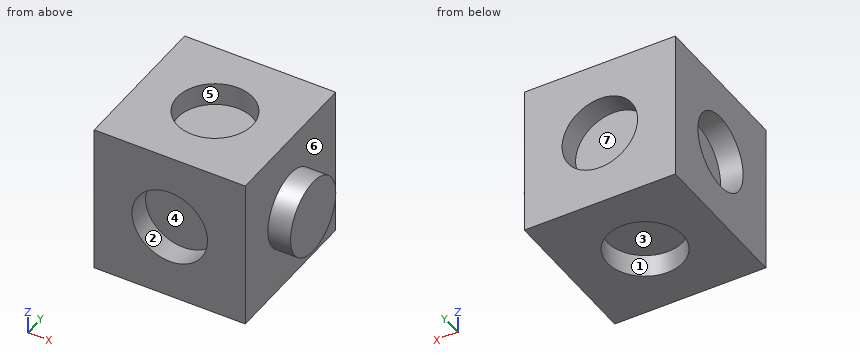
```python
from build123d import *

# Parameters (mm, degrees)
F0_W      = 25.4
F0_H      = 25.4
F1_DEPTH  = 25.4
F7_R      = 6.35
F8_DEPTH  = 3.81
F6_R      = 6.35
F9_DEPTH  = 3.81
F5_R      = 6.35
F10_DEPTH = 3.81
F4_R      = 6.35
F11_DEPTH = 3.81
F3_R      = 6.35
F12_DEPTH = 3.81
F2_R      = 6.35
F13_DEPTH = 3.81


with BuildPart() as f1:
    # F0 (on Front) → F1 (new body)
    with BuildSketch(Plane.XZ):
        with Locations((5.750718, -12.019807)):
            Rectangle(F0_W, F0_H)
    extrude(amount=F1_DEPTH)

    # F7 (on face) → F8 (cut)
    with BuildSketch(Plane(origin=(0, 0, 0), x_dir=(-1, 0, 0), z_dir=(0, 1, 0))):
        with Locations((-5.750718, -12.019807)):
            Circle(F7_R)
    extrude(amount=-F8_DEPTH, mode=Mode.SUBTRACT)

    # F6 (on face) → F9 (cut)
    with BuildSketch(Plane(origin=(-6.949282, 0, 0), x_dir=(0, -1, 0), z_dir=(-1, 0, 0))):
        with Locations((12.7, -12.019807)):
            Circle(F6_R)
    extrude(amount=-F9_DEPTH, mode=Mode.SUBTRACT)

    # F5 (on face) → F10 (cut)
    with BuildSketch(Plane.XY.offset(0.680193)):
        with Locations((5.75072, -12.7)):
            Circle(F5_R)
    extrude(amount=-F10_DEPTH, mode=Mode.SUBTRACT)

    # F4 (on face) → F11 (join)
    with BuildSketch(Plane.YZ.offset(18.450718)):
        with Locations((-12.7, -12.019807)):
            Circle(F4_R)
    extrude(amount=F11_DEPTH)

    # F3 (on face) → F12 (cut)
    with BuildSketch(Plane(origin=(0, 0, -24.719807), x_dir=(1, 0, 0), z_dir=(0, 0, -1))):
        with Locations((5.750718, 12.7)):
            Circle(F3_R)
    extrude(amount=-F12_DEPTH, mode=Mode.SUBTRACT)

    # F2 (on face) → F13 (cut)
    with BuildSketch(Plane.XZ.offset(25.4)):
        with Locations((5.750718, -12.019807)):
            Circle(F2_R)
    extrude(amount=-F13_DEPTH, mode=Mode.SUBTRACT)


solid = f1.part
```
The listing builds one solid part. Answer for the finished solid, in the listing's coordinates (mm). Face numbers are marked on the shaded views. A direction names the side the tool comes from. Give positions to 0.01 mm unless a question says otherwise; leave off trailing zeros. Order: outer loops, then holes, each group sorted by start corner. A loop starts at its lowest first (then second) coordinate and runs counter-clockwise, first axis right, second up. Notation, with made-up numbers: (87.5, -21.75) -> (107.5, -21.75) arc R21 cw to (107.5, 14.25) -> close; hole circle Ø7 at (-18.5, 38.5). An arc over 180 degrees is marked (long way). One line per item, written item: value.
1) Find section A-A, the plane y = -12.7. Determine the outline of the cut face in (x, z), plus the area to 3 significant figures.
Reported:
outline: (-6.95, -24.72) -> (-0.6, -24.72) -> (-0.6, -20.91) -> (12.1, -20.91) -> (12.1, -24.72) -> (18.45, -24.72) -> (18.45, -18.37) -> (22.26, -18.37) -> (22.26, -5.67) -> (18.45, -5.67) -> (18.45, 0.68) -> (12.1, 0.68) -> (12.1, -3.13) -> (-0.6, -3.13) -> (-0.6, 0.68) -> (-6.95, 0.68) -> (-6.95, -5.67) -> (-3.14, -5.67) -> (-3.14, -18.37) -> (-6.95, -18.37) -> close
area: 548 mm^2
2) Find section D-D, the plane y = -4.75. Determine the outline of the cut face in (x, z).
Reported:
outline: (-6.95, -24.72) -> (18.45, -24.72) -> (18.45, 0.68) -> (-6.95, 0.68) -> close
3) Determine the mould class of the marked faces 1, 2, 3 and 4 for opening direction Z: pulls with the +Z half, pulls with the -Z half, needs draft (parallel to the pull), parting line crosses it, or undercut.
Reported:
face 1: needs draft
face 2: undercut
face 3: pulls with the -Z half
face 4: undercut
4) Find section B-B, the plane z = -7.5. Determine the outline of the cut face in (x, y).
Reported:
outline: (-6.95, -25.4) -> (1.29, -25.4) -> (1.29, -21.59) -> (10.21, -21.59) -> (10.21, -25.4) -> (18.45, -25.4) -> (18.45, -17.16) -> (22.26, -17.16) -> (22.26, -8.24) -> (18.45, -8.24) -> (18.45, 0) -> (10.21, 0) -> (10.21, -3.81) -> (1.29, -3.81) -> (1.29, 0) -> (-6.95, 0) -> (-6.95, -8.24) -> (-3.14, -8.24) -> (-3.14, -17.16) -> (-6.95, -17.16) -> close
5) A tool of negligible diameter and unlimited length cuts with its end or side. For the marked faces 5, 6 and 7, from which of +Z, -Z, +X, -X, +Y, -Y can it reach the whole face along a straight path? Write none if from no direction.
Reported:
face 5: +Z
face 6: +X
face 7: +Y
6) Find section C-C, the plane y = -2. Determine the outline of the cut face in (x, z), plus the area to 3 significant figures.
Reported:
outline: (-6.95, -24.72) -> (18.45, -24.72) -> (18.45, 0.68) -> (-6.95, 0.68) -> close; hole circle Ø12.7 at (5.75, -12.02)
area: 518 mm^2
7) Find the intervals of material crossed by line 1 (Z direction, x = -5.5, y = -12.7); line 2 (X direction, y = -11.5, z = -10); line 3 (X direction, y = -15.5, z = -5), in increasing order.
Reported:
line 1: z = -24.72 to -18.37, -5.67 to 0.68
line 2: x = -3.14 to 22.26
line 3: x = -6.95 to 18.45
8) Flat-ended cylindrical pins translate along their axes: P1, Ø10, axis at x = 5, y = -11, coming from the +Z side; P2, Ø1.5, axis at y = -6.5, z = -3.5, coming from the +X side; P3, Ø11.5, axis at x = 5.75, y = -12.7, coming from the -Z side; P4, Ø1, axis at x = 7, z = -6.5, coming from the -Y side. Find the tip coordinate at first contact, or state that the pin passes through.
Reported:
P1: stops at z = 0.68
P2: stops at x = 18.45
P3: stops at z = -20.91
P4: stops at y = -21.59
